Read the model definition and answer for the solid it produces. Units are mm, in the model's axes. A direction names the side the tool comes from. Coordinates: 2 decimals unless noted, no trailing zeros. Loops run counter-clockwise (first coordinate to the right, second up) from the corner with the lowest first, then second, coordinate; pieces in that order, holes last. Notation, with made-up numbers: (63, -33) -> (115, -33) arc R27 ccw to (115, -8) -> close; hole circle Ø3 at (82.25, -34.75). An arc over 180 degrees is marked (long way). Answer as a JSON object with one key per item and string values. Group by question number.
1) Section C-C, the plane x = 1.2 is taken. Count the separate pieces of the cut face and the enclosed holes in it, plus the area to 3 significant figures.
2) Section A-A, the plane z = 0 is taken. Give the vertices of the cut face in (x, y).
3) Section B-B, the plane y = -14 is taken. Give the vertices of the cut face in (x, z).
4) Consider probe 1 along Z at (x, y) = (2.45, -15); probe 2 along Z at (x, y) = (1.4, -53.5); probe 3 along Y at (x, z) = (1.15, -37). Determine where each line is inside the solid, lowest interval first. Write a range as [from, to].
5) Section D-D, the plane z = -33.5 is taken. Give the vertices of the cut face in (x, y), plus the area to 3 significant figures.
6) Which of the six approach directions +Z, -Z, +X, -X, +Y, -Y give full straight-line access (tool end or side, diameter ignored) to faces 5 (the face through (1.479, -3.523, 37.735)), 6 (the face through (1.479, -62.137, -53.825)), 7 (the face through (1.48, 21.46, 32.71))?
7) Determine the mould class of faces 1 (the face through (1.479, -62.023, 53.844)), 2 (the face through (1.48, -43.83, 53.71)), 3 (the face through (1.479, 4.713, 28.341)), 4 (the face through (3, -3, 4)) for opening direction Y: released by +Y, released by -Y, zero draft, split by the parting line, or undercut.
8) Flat-ended cylindrical pins translate along their axes: P1, Ø4, axis at y = 0, z = 0, coming from the -X side; P2, Ø1.5, axis at x = 2.5, z = 49, coming from the -Y side; P3, Ø1, axis at x = 1.5, y = -48, coming from the +Z side. Find the tip coordinate at first contact, or state that the pin passes through.
from build123d import *

# Parameters (mm, degrees)
SKETCH1_R           = 3.45
SKETCH1_R_2         = 1.05
BOSS_EXTRUDE1_DEPTH = 3


with BuildPart() as part:
    # Sketch1 → Boss-Extrude1 (new body)
    with BuildSketch(Plane(origin=(0, 0, 0), x_dir=(0, 0, -1), z_dir=(1, 0, 0))):
        with BuildLine():
            Line((1.710100717, 11.072425758), (29.81221294, 21.300758128))
            ThreePointArc((29.81221294, 21.300758128), (32.665838041, 21.469774041), (35.145679665, 20.04775853))
            Line((35.145679665, 20.04775853), (54.503522355, -0.309603856))
            Line((54.503522355, -0.309603856), (64.462541824, -28.342275903))
            Line((64.462541824, -28.342275903), (62.158643896, -58.002094263))
            Line((62.158643896, -58.002094263), (57.918218143, -67.574774191))
            ThreePointArc((57.918218143, -67.574774191), (54.918016136, -68.957985447), (53.165427908, -66.157464075))
            Line((53.165427908, -66.157464075), (54.503522355, -58.002094263))
            Line((54.503522355, -58.002094263), (52.939962821, -30.04554677))
            Line((52.939962821, -30.04554677), (44.360806264, -10.45))
            Line((44.360806264, -10.45), (31.292334945, 3.213047447))
            ThreePointArc((31.292334945, 3.213047447), (28.386766522, 4.706668614), (25.179055571, 4.087134512))
            Line((25.179055571, 4.087134512), (2.5, -9.006624327))
            ThreePointArc((2.5, -9.006624327), (0, -9.676497308), (-2.5, -9.006624327))
            Line((-2.5, -9.006624327), (-25.179055571, 4.087134512))
            ThreePointArc((-25.179055571, 4.087134512), (-28.386766522, 4.706668614), (-31.292334945, 3.213047447))
            Line((-31.292334945, 3.213047447), (-44.360806264, -10.45))
            Line((-44.360806264, -10.45), (-52.939962821, -30.04554677))
            Line((-52.939962821, -30.04554677), (-54.503522355, -58.002094263))
            Line((-54.503522355, -58.002094263), (-53.165427908, -66.157464075))
            ThreePointArc((-53.165427908, -66.157464075), (-54.918016136, -68.957985447), (-57.918218143, -67.574774191))
            Line((-57.918218143, -67.574774191), (-62.158643896, -58.002094263))
            Line((-62.158643896, -58.002094263), (-64.462541824, -28.342275903))
            Line((-64.462541824, -28.342275903), (-54.503522355, -0.309603856))
            Line((-54.503522355, -0.309603856), (-35.145679665, 20.04775853))
            ThreePointArc((-35.145679665, 20.04775853), (-32.665838041, 21.469774041), (-29.81221294, 21.300758128))
            Line((-29.81221294, 21.300758128), (-1.710100717, 11.072425758))
            ThreePointArc((-1.710100717, 11.072425758), (0, 10.770888862), (1.710100717, 11.072425758))
        make_face()
        Circle(SKETCH1_R, mode=Mode.SUBTRACT)
        with Locations((13.357740048, 5.51119595)):
            Circle(SKETCH1_R_2, mode=Mode.SUBTRACT)
    extrude(amount=BOSS_EXTRUDE1_DEPTH)


solid = part.part
Determined:
{
 "1": {"separate pieces": "1", "enclosed holes": "2", "area": "3,130 mm²"},
 "2": {"outline": "(0, -9.68) -> (3, -9.68) -> (3, -3.45) -> (0, -3.45) -> close; (0, 3.45) -> (3, 3.45) -> (3, 10.77) -> (0, 10.77) -> close"},
 "3": {"outline": "(0, -59.37) -> (3, -59.37) -> (3, -45.92) -> (0, -45.92) -> close; (0, 45.92) -> (3, 45.92) -> (3, 59.37) -> (0, 59.37) -> close"},
 "4": {"probe 1": "[-59.72, -46.35], [46.35, 59.72]", "probe 2": "[-62.51, -54.25], [54.25, 62.51]", "probe 3": "[-2.75, 18.1]"},
 "5": {"outline": "(0, 0.9) -> (3, 0.9) -> (3, 21.19) -> (0, 21.19) -> close", "area": "60.9 mm²"},
 "6": {"face 5": "+X, -X, -Y", "face 6": "+X, -X", "face 7": "+X, -X, +Y"},
 "7": {"face 1": "undercut", "face 2": "undercut", "face 3": "released by -Y", "face 4": "zero draft"},
 "8": {"P1": "through", "P2": "y = -22.76", "P3": "z = 62.97"}
}
